Geometry check sheet. Reference: the model listing, model coordinates, mm. Face numbers are marked on the shaded views. Coordinates: 2 decimals unless noted, no trailing zeros. Loops run counter-clockwise (first coordinate to the right, second up) from the corner with the lowest first, then second, coordinate; pieces in that order, holes last. Notation, with made-up numbers: (-37, -26.5) - (-9, -26.5) arc R23 ccw to (-9, -7.5) - close; hole circle Ø2 at (73, 84.25). An arc over 180 degrees is marked (long way). One line per item, written item: value.
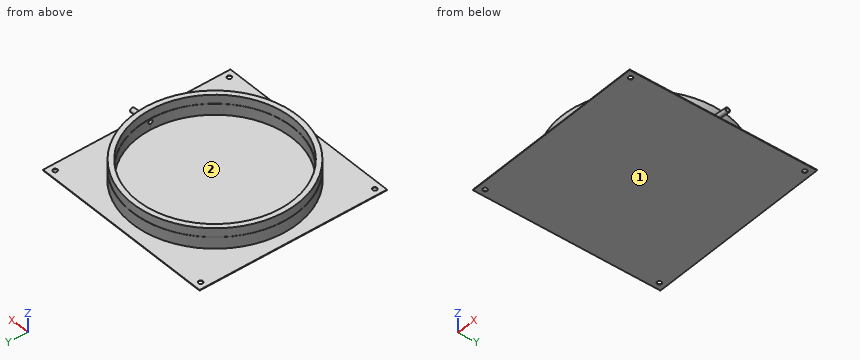
from build123d import *
from build123d import SkipClean  # not in build123d's __all__

# Parameters (mm, degrees)
F0_W     = 10
F0_H     = 3
F2_W     = 850
F2_H     = 850
F2_R     = 10
F3_DEPTH = 3
F6_R     = 9
F7_DEPTH = 120
F8_R     = 350
F9_DEPTH = 200


with BuildPart() as f1:
    # F0 (on Front) → F1 (revolve)
    with BuildSketch(Plane.XZ):
        Polygon((-375, 5), (-350, 5), (-350, 55), (-351, 55), (-351, 95), (-374, 95), (-374, 55), (-375, 55), align=None)
        Polygon((-10, 5), (-350, 5), (-375, 5), (-375, 2), (-10, 2), align=None)
        with Locations((-5, 3.5)):
            Rectangle(F0_W, F0_H)
    revolve(axis=Axis((0, 0, 187.9212413023), (0, 0, -1)))

    # F2 (on Top) → F3 (join)
    with BuildSketch(Plane.XY):
        Rectangle(F2_W, F2_H)
        with Locations((-395, -395)):
            Circle(F2_R, mode=Mode.SUBTRACT)
        with Locations((395, -395)):
            Circle(F2_R, mode=Mode.SUBTRACT)
        with Locations((-395, 395)):
            Circle(F2_R, mode=Mode.SUBTRACT)
        with Locations((395, 395)):
            Circle(F2_R, mode=Mode.SUBTRACT)
    extrude(amount=F3_DEPTH)

    # F4 (on Front) → F5 (revolve)
    with BuildSketch(Plane.XZ):
        Polygon((449.6194698092, 41.5098406888), (350, 50.2254149636), (349.9128442573, 49.2292202655), (449.5323140664, 40.5136459907), align=None)
    revolve(axis=Axis((462.7442754949, 0, 30.3233706049), (0.9961946981, 0, -0.0871557427)))

    # F6 (on face) → F7 (cut)
    with BuildSketch(Plane(origin=(442.6000506958, 0, -38.7224869119), x_dir=(0, 1, 0), z_dir=(0.9961946981, 0, -0.0871557427))):
        with Locations((0, 70.5388020579)):
            Circle(F6_R)
    extrude(amount=-F7_DEPTH, mode=Mode.SUBTRACT)

    # F8 (on face) → F9 (cut)
    with BuildSketch(Plane.XY.offset(5)):
        Circle(F8_R)
    with SkipClean():  # cleaning this boolean's faces spoils the solid; the shape is the same uncleaned
        extrude(amount=F9_DEPTH, mode=Mode.SUBTRACT)


solid = f1.part
(1) Material ranges on probe 1 along Y at (x, z) = (-395, 1); probe 2 along Y at (x, z) = (0, 76); probe 3 along X at (y, z) = (-6, 81), recorded low to high. Write a range as from..to.
Reply:
probe 1: -425..-405, -385..385, 405..425
probe 2: -374..-351, 351..374
probe 3: -373.95..-350.95, 350.95..373.95
(2) Go/stop test with flat-tipped pins: pin 1 Ø1 at (x, z) = (175, 70) entering from +Y; pin 2 Ø5 at (x, z) = (318.5, 20) entering from -Y; pin 3 Ø8 at (x, y) = (237.5, -121) entering from +Z. Record where each tip stops, or that it passes through.
Reply:
pin 1: y = 330.8
pin 2: y = -201.91
pin 3: z = 5
(3) Release check for a two-part mould opening along Y. For the marked faces 1 and 2 record: pulls with the +Y half, pulls with the -Y half, needs draft (parallel to the pull), parting line crosses it, or undercut.
Reply:
face 1: needs draft
face 2: undercut
(4) Cross-section at A-A on x = -395. Record the cut outline in (y, z).
Reply:
outline: (-425, 0) - (-405, 0) - (-405, 3) - (-425, 3) - close; (-385, 0) - (385, 0) - (385, 3) - (-385, 3) - close; (405, 0) - (425, 0) - (425, 3) - (405, 3) - close
(5) Cross-section at D-D on y = 63. Record the cut outline in (x, z).
Reply:
outline: (-425, 0) - (425, 0) - (425, 3) - (369.67, 3) - (369.67, 55) - (368.66, 55) - (368.66, 95) - (345.3, 95) - (345.3, 55) - (344.28, 55) - (344.28, 5) - (-344.28, 5) - (-344.28, 55) - (-345.3, 55) - (-345.3, 95) - (-368.66, 95) - (-368.66, 55) - (-369.67, 55) - (-369.67, 3) - (-425, 3) - close
(6) Cross-section at C-C on x = 0. Record the cut outline in (y, z).
Reply:
outline: (-425, 0) - (425, 0) - (425, 3) - (375, 3) - (375, 55) - (374, 55) - (374, 95) - (351, 95) - (351, 55) - (350, 55) - (350, 5) - (-350, 5) - (-350, 55) - (-351, 55) - (-351, 95) - (-374, 95) - (-374, 55) - (-375, 55) - (-375, 3) - (-425, 3) - close
